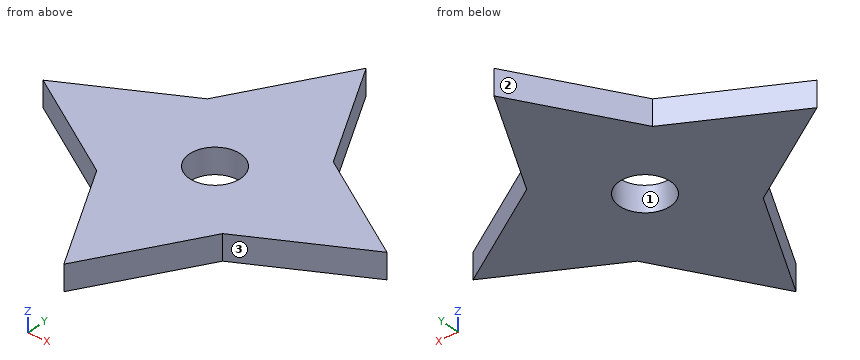
```python
from build123d import *

# Parameters (mm, degrees)
F0_W          = 50
F0_H          = 50
F1_DEPTH      = 5
F1_DEPTH_BACK = 5
F2_R          = 10
F3_DEPTH      = 10.001


with BuildPart() as f1:
    # F0 (on Top) → F1 (new body, two sides)
    with BuildSketch(Plane.XY) as f1_sk:
        Rectangle(F0_W, F0_H)
        Polygon((68.3012701892, 0), (25, 25), (25, -25), align=None)
        Polygon((-25, 25), (25, 25), (0, 68.3012701892), align=None)
        Polygon((-25, -25), (-25, 25), (-68.3012701892, 0), align=None)
        Polygon((0, -68.3012701892), (25, -25), (-25, -25), align=None)
    extrude(amount=F1_DEPTH)
    extrude(f1_sk.sketch, amount=-F1_DEPTH_BACK)

    # F2 (on face) → F3 (cut, through all)
    with BuildSketch(Plane.XY.offset(5)):
        Circle(F2_R)
    extrude(amount=-F3_DEPTH, mode=Mode.SUBTRACT)


solid = f1.part
```
The listing builds one solid part. Answer for the finished solid, in the listing's coordinates (mm). Face numbers are marked on the shaded views. Coordinates: 2 decimals unless noted, no trailing zeros. Loops run counter-clockwise (first coordinate to the right, second up) from the corner with the lowest first, then second, coordinate; pieces in that order, holes last. Notation, with made-up numbers: (56, 82) -> (82, 82) arc R18 cw to (82, 102) -> close; hole circle Ø6 at (-16, 44). An arc over 180 degrees is marked (long way). Use one line per item in the form item = value. Start each with the question number.
Item 1: Flat-ended cylindrical pins translate along their axes: pin 1 Ø2 at (x, z) = (-47, 3) entering from -Y; pin 2 Ø4 at (x, z) = (50.5, -1.5) entering from -Y. Find the tip coordinate at first contact, or state that the pin passes through.
Item 2: The part is cut by section C-C on y = -32. Determine the outline of the cut face in (x, z).
Item 3: The part is cut by section A-A on z = 1.75. Determine the outline of the cut face in (x, y), then the cut area to 3 significant figures.
Item 4: Consider L1, parallel to Y at x = 0, z = -1.5; L2, parallel to X at y = 2.5, z = 4.5; L3, parallel to Y at x = -3, z = 1. Determine where each line is inside the solid, lowest interval first. Write a range as [from, to].
Item 5: The part is cut by section B-B on x = -36. Determine the outline of the cut face in (y, z), then the cut area to 3 significant figures.
Item 6: The mould has two halves that part along Y. Classify the marked faces 1, 2 and 3: released by +Y, released by -Y, zero draft, split by the parting line, or undercut.
Answer key:
q1.pin_1 = -12.88
q1.pin_2 = -11.43
q2.outline = (-20.96, -5) -> (20.96, -5) -> (20.96, 5) -> (-20.96, 5) -> close
q3.outline = (-68.3, 0) -> (-25, -25) -> (0, -68.3) -> (25, -25) -> (68.3, 0) -> (25, 25) -> (0, 68.3) -> (-25, 25) -> close; hole circle Ø20 at (0, 0)
q3.area = 6,520 mm2
q4.L1 = [-68.3, -10], [10, 68.3]
q4.L2 = [-63.97, -9.68], [9.68, 63.97]
q4.L3 = [-63.11, -9.54], [9.54, 63.11]
q5.outline = (-18.65, -5) -> (18.65, -5) -> (18.65, 5) -> (-18.65, 5) -> close
q5.area = 373 mm2
q6.face_1 = undercut
q6.face_2 = released by +Y
q6.face_3 = released by -Y
